Geometry check sheet. Reference: the model listing, model coordinates, mm. A direction names the side the tool comes from. Round coordinates to 2 decimals unless told otherwise and drop trailing zeros. Write each loop counter-clockwise with the first axis right and the second up, starting at its lowest first coordinate (ties: lowest second). Pieces come first, ordered by that corner, then holes.
Item 1: Draft check along Y on faces 5 (the face through (-9, 6, 7.4)), 6 (the face through (-4, 34.5, 6)), 7 (the face through (-0.807, 0.051, 3.752)). Enter one of: pulls with the +Y half, pulls with the -Y half, needs draft (parallel to the pull), parting line crosses it, or undercut.
Item 2: Cross-section at C-C (x = 1). Enter the section's corners in (y, z), then the cut area to 3 significant figures.
Item 3: Cross-section at A-A (x = -3.75). Enter the section's corners in (y, z), then the cut area to 3 significant figures.
Item 4: Access from +Z, -Z, +X, -X, +Y, -Y to the whole of each face (thin tool, end or side, straight path). Record for faces 1 (the face through (-1.092, 7, 4)), 2 (the face through (-8.215, -22.199, 2.535)), 3 (the face through (8.5, 29, 6)), 4 (the face through (-13, 13, 5)).
Item 5: Cross-section at B-B (z = 1). Enter the section's corners in (x, y), then the cut area to 3 significant figures.
Item 6: Cross-section at D-D (y = -6.5). Enter the section's corners in (x, z).
Item 7: Scan lines: probe 1 along X at (y, z) = (-14, 0.75); probe 2 along X at (y, z) = (11.5, 1); probe 3 along Y at (x, z) = (-5.5, 7.25). Record each from-to range of solid material in increasing order.
Item 8: Depth check by flat-ended pin: P1, Ø0.7, axis at y = 17, z = 6, coming from the +X side; P2, Ø3, axis at y = 3, z = 1, coming from the +X side; P3, Ø1, axis at x = -6.5, z = 1.5, coming from the +Y side. Enter the tip coordinate at first touch or a pass-through.
from build123d import *

# Parameters (mm, degrees)
SKETCH1_W           = 17
SKETCH1_H           = 45
BOSS_EXTRUDE1_DEPTH = 12
BOSS_EXTRUDE2_DEPTH = 7
FILLET1_R           = 4
CUT_EXTRUDE1_DEPTH  = 42.886752082
CUT_EXTRUDE2_START  = -4.6
CUT_EXTRUDE2_DEPTH  = 4.6
SKETCH5_W           = 8
SKETCH5_H           = 8
CUT_EXTRUDE3_DEPTH  = 41.807597332
FILLET2_R           = 1
FILLET3_R           = 1


with BuildPart() as part:
    # Sketch1 → Boss-Extrude1 (new body)
    with BuildSketch(Plane.XY):
        Rectangle(SKETCH1_W, SKETCH1_H)
    extrude(amount=BOSS_EXTRUDE1_DEPTH)

    # Sketch2 → Boss-Extrude2 (add)
    with BuildSketch(Plane.XY.offset(12)):
        Polygon((-8.5, -22.5), (-8.5, 22.5), (8.5, 22.5), (8.5, 34.5), (-20.5, 34.5), (-20.5, -22.5), align=None)
    extrude(amount=-BOSS_EXTRUDE2_DEPTH)

    # Fillet1
    fillet1_edges = [part.edges().sort_by_distance(p)[0] for p in [
        (-20.5, 34.5, 8.5),
    ]]
    fillet(fillet1_edges, radius=FILLET1_R)

    # Sketch3 → Cut-Extrude1 (cut, through all)
    with BuildSketch(Plane(origin=(0, 0, 0), x_dir=(-1, 0, 0), z_dir=(0, 0, -1))):
        Polygon((-2.5, -0.25), (1.091673087, -0.25), (1.091673087, 22.5), (-8.5, 22.5), (-8.5, -0.25), (-3.5, -0.25), align=None)
    extrude(amount=-CUT_EXTRUDE1_DEPTH, mode=Mode.SUBTRACT)

    # Sketch4 → Cut-Extrude2 (cut)
    with BuildSketch(Plane.XY.offset(12).offset(CUT_EXTRUDE2_START)):
        with BuildLine():
            Line((-1.091673087, -0.25), (-1.091673087, 22.5))
            Line((-1.091673087, 22.5), (8.5, 22.5))
            Line((8.5, 22.5), (8.5, 34.5))
            Line((8.5, 34.5), (-16.5, 34.5))
            ThreePointArc((-16.5, 34.5), (-19.328427125, 33.328427125), (-20.5, 30.5))
            Line((-20.5, 30.5), (-20.5, -22.5))
            Line((-20.5, -22.5), (8.5, -22.5))
            Line((8.5, -22.5), (8.5, -0.25))
            Line((8.5, -0.25), (-1.091673087, -0.25))
        make_face()
    extrude(amount=CUT_EXTRUDE2_DEPTH, mode=Mode.SUBTRACT)

    # Sketch5 → Cut-Extrude3 (cut, through all)
    with BuildSketch(Plane(origin=(0, 0, 0), x_dir=(-1, 0, 0), z_dir=(0, 0, -1))):
        with Locations((4.5, 18.5)):
            Rectangle(SKETCH5_W, SKETCH5_H)
    extrude(amount=-CUT_EXTRUDE3_DEPTH, mode=Mode.SUBTRACT)

    # Fillet2
    fillet2_edges = [part.edges().sort_by_distance(p)[0] for p in [
        (-8.5, 22.5, 6.2),
        (-8.5, 14.5, 6.2),
        (-1.091673087, 14.5, 3.7),
        (-1.091673087, -0.25, 3.7),
        (8.5, -0.25, 3.7),
        (8.5, 22.5, 6.2),
    ]]
    fillet(fillet2_edges, radius=FILLET2_R)

    # Fillet3
    fillet3_edges = [part.edges().sort_by_distance(p)[0] for p in [
        (-8.5, -22.5, 2.5),
        (-8.5, 14.5, 2.5),
    ]]
    fillet(fillet3_edges, radius=FILLET3_R)


solid = part.part
Resolved:
1. face 5: needs draft
1. face 6: pulls with the +Y half
1. face 7: undercut
2. outline: (-22.5, 0) - (-0.25, 0) - (-0.25, 7.4) - (-22.5, 7.4) - close; (22.5, 5) - (34.5, 5) - (34.5, 7.4) - (22.5, 7.4) - close
2. area: 193 mm2
3. outline: (-22.5, 0) - (14.5, 0) - (14.5, 7.4) - (-22.5, 7.4) - close; (22.5, 5) - (34.5, 5) - (34.5, 7.4) - (22.5, 7.4) - close
3. area: 303 mm2
4. face 1: +Z, -Z, +X
4. face 2: -Z, -X, -Y
4. face 3: +Z, -Z, +X, +Y, -Y
4. face 4: -Z, -X, +Y
5. outline: (-8.5, -21.5) arc R1 ccw to (-7.5, -22.5) - (8.5, -22.5) - (8.5, -1.25) arc R1 ccw to (7.5, -0.25) - (-0.09, -0.25) arc R1 cw to (-1.09, 0.75) - (-1.09, 13.5) arc R1 ccw to (-2.09, 14.5) - (-7.5, 14.5) arc R1 ccw to (-8.5, 13.5) - close
5. area: 487 mm2
6. outline: (-20.5, 5) - (-8.5, 5) - (-8.5, 0) - (8.5, 0) - (8.5, 7.4) - (-20.5, 7.4) - close
7. probe 1: x = -8.5 to 8.5
7. probe 2: x = -8.5 to -1.09
7. probe 3: y = -22.5 to 14.5, 22.5 to 34.5
8. P1: stops at x = -8.5
8. P2: stops at x = -1.09
8. P3: stops at y = 14.5
